```python
from build123d import *

# Parameters (mm, degrees)
F0_W        = 111.125
F0_H        = 7.3025
F0_R        = 0.635
F1_DEPTH    = 1.5875
F2_R        = 3.5566194201
F3_T1_DEPTH = 20.2904124677


# Not quite as in the source:
# - a fillet or chamfer that OpenCascade refuses, or shapes differently, is made with other operations: its cross-section is extruded or revolved along the edge and cut away or added


with BuildPart() as f1:
    # F0 (on Front) → F1 (new body)
    with BuildSketch(Plane.XZ):
        with Locations((8.7715025485, 10.1259618964)):
            Rectangle(F0_W, F0_H)
        with Locations((-43.7429974515, 10.1259618964)):
            Circle(F0_R, mode=Mode.SUBTRACT)
        with Locations((61.2860025485, 10.1196118964)):
            Circle(F0_R, mode=Mode.SUBTRACT)
    extrude(amount=F1_DEPTH)

    # F2
    f2_edges = [f1.edges().sort_by_distance(p)[0] for p in [
        (-46.790997, -0.79375, 13.777212),
        (-46.790997, -0.79375, 6.474712),
    ]]
    fillet(f2_edges, radius=F2_R)

    # F3: fillet of radius 3.7405824935 on 2 edges, made by hand

    # F3_s2 → F3_t1 (cut)
    with BuildSketch(Plane.XZ.offset(-9.3514562339)):
        with BuildLine():
            ThreePointArc((60.5934200549, 13.7772118964), (63.2384113017, 12.6816206496), (64.3340025485, 10.0366294028))
            Line((64.3340025485, 10.0366294028), (64.3340025485, 13.7772118964))
            Line((64.3340025485, 13.7772118964), (60.5934200549, 13.7772118964))
        make_face()
        with BuildLine():
            ThreePointArc((64.3340025485, 10.2152943899), (63.2384113017, 7.5703031432), (60.5934200549, 6.4747118964))
            Line((60.5934200549, 6.4747118964), (64.3340025485, 6.4747118964))
            Line((64.3340025485, 6.4747118964), (64.3340025485, 10.2152943899))
        make_face()
    extrude(amount=F3_T1_DEPTH, mode=Mode.SUBTRACT)


solid = f1.part
```
Work out the finished part from the listing and answer in its coordinate system (mm). Round coordinates to 2 decimals unless told otherwise and drop trailing zeros. Write each loop counter-clockwise with the first axis right and the second up, starting at its lowest first coordinate (ties: lowest second). Pieces come first, ordered by that corner, then holes.
1) A cutting plane is placed at A-A on y = -0.25. Determine the outline of the cut face in (x, z) (3 decimals), and give its area (3 significant figures).
2) Consider probe 1 along X at (y, z) = (-1.25, 10.25); probe 2 along X at (y, z) = (-1.2, 9.75); probe 3 along X at (y, z) = (-0.1, 11.75). Determine where each line is inside the solid, lowest interval first.
3) A cutting plane is placed at B-B on z = 7.5. Determine the outline of the cut face in (x, y), and give its area (3 significant figures).
Entries:
1. outline: (-46.791, 10.031) arc R3.557 ccw to (-43.234, 6.475) - (60.593, 6.475) arc R3.741 ccw to (64.333, 10.126) arc R3.741 ccw to (60.593, 13.777) - (-43.234, 13.777) arc R3.557 ccw to (-46.791, 10.221) - close; hole circle Ø1.27 at (-43.743, 10.126); hole circle Ø1.27 at (61.286, 10.12)
1. area: 798 mm2
2. probe 1: x = -46.79 to -44.37, -43.12 to 60.66, 61.91 to 64.33
2. probe 2: x = -46.78 to -44.25, -43.23 to 60.77, 61.8 to 64.3
2. probe 3: x = -46.45 to 63.92
3. outline: (-45.73, -1.59) - (63.17, -1.59) - (63.17, 0) - (-45.73, 0) - close
3. area: 173 mm2
